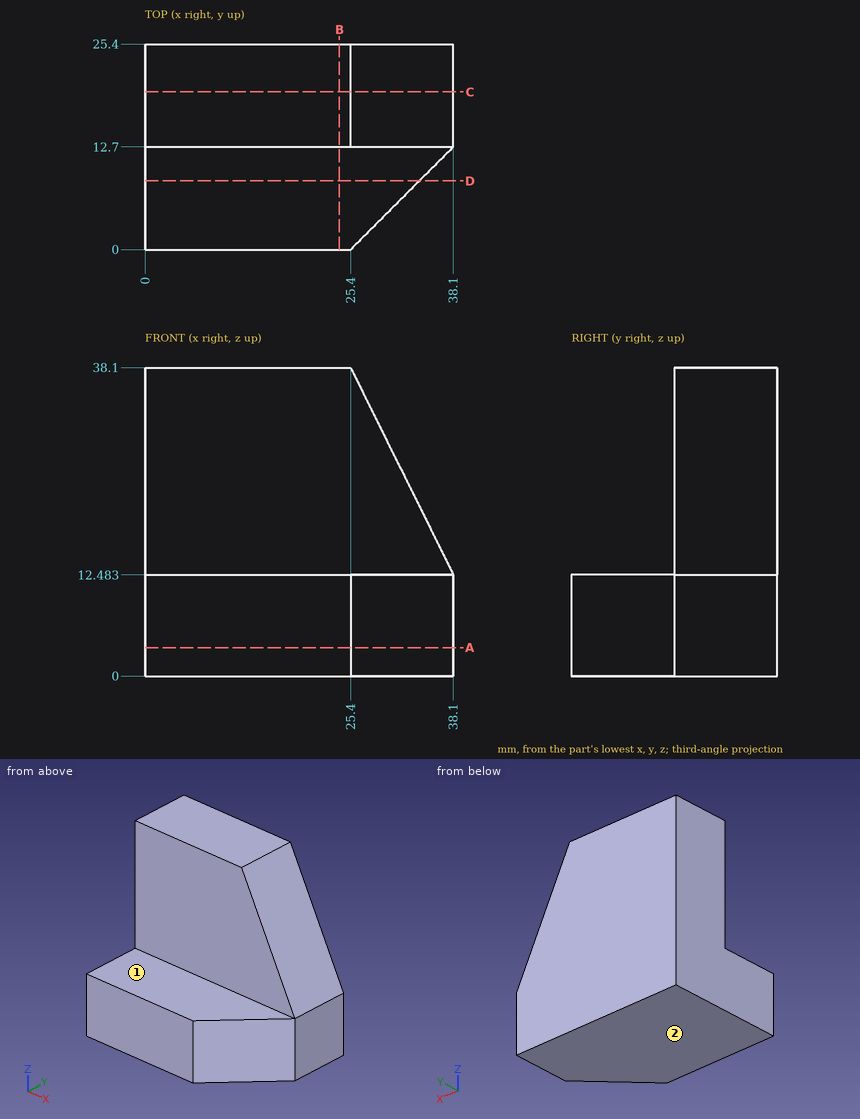
Design review of the part shown in the three views and the two pictorial views. Dimensions are in mm from the part's minimum x, y and z. A direction names the side the tool comes from. Give positions to 0.01 mm unless a question says otherwise; leave off trailing zeros. Loops run counter-clockwise (first coordinate to the right, second up) from the corner with the lowest first, then second, coordinate; pieces in that order, holes last. Notation, with made-up numbers: M -36.5,32 L -19.5,32 A11 cw -19.5,51 Z; hole C 28.25,78 d10. An arc over 180 degrees is marked long. Answer as a JSON object with one key per item and string values. Group by question number.
Q1. Add section D-D on y = 8.5. Give the boundary of the cut face in (x, z).
Q2. Tool access review of the marked faces 1 and 2: name each direction out of +Z, -Z, +X, -X, +Y, -Y from which nothing blocks a thin tool from reaching the whole face with its end or side.
Q3. Add section C-C on y = 19.5. Give the boundary of the cut face in (x, z).
Q4. Add section A-A on z = 3.5. Give the boundary of the cut face in (x, y).
Q5. For probe 1 along Z at (x, y) = (5, 12.25); probe 2 along Y at (x, z) = (10.5, 22.5); probe 3 along X at (y, z) = (20, 32.5), list the stretches that pass through material, from the lowest coordinate up. Write a range as [from, to].
Q6. Add section B-B on x = 24. Give the boundary of the cut face in (y, z).
Q7. Insertion check: P1, Ø10, axis at x = 32.5, y = 10.5, coming from the +Z side (1 decimal); P2, Ø7.5, axis at x = 18, z = 26, coming from the -Y side; P3, Ø4, axis at x = 27.5, y = 8.5, coming from the +Z side. Each pin has a flat end and moves straight along its axis. Give the tip position at first contact, or say it passes through.
Checked values:
{
 "1": {"outline": "M 0,0 L 33.9,0 L 33.9,12.48 L 0,12.48 Z"},
 "2": {"face 1": "+Z, +X, -X, -Y", "face 2": "-Z, +X, -X, +Y, -Y"},
 "3": {"outline": "M 0,0 L 38.1,0 L 38.1,12.48 L 25.4,38.1 L 0,38.1 Z"},
 "4": {"outline": "M 0,0 L 25.4,0 L 38.1,12.7 L 38.1,25.4 L 0,25.4 Z"},
 "5": {"probe 1": "[0, 12.48]", "probe 2": "[12.7, 25.4]", "probe 3": "[0, 28.18]"},
 "6": {"outline": "M 0,0 L 25.4,0 L 25.4,38.1 L 12.7,38.1 L 12.7,12.48 L 0,12.48 Z"},
 "7": {"P1": "z = 32.8", "P2": "y = 12.7", "P3": "z = 12.48"}
}
